Geometry: final body of the model. Coordinates: model frame, mm. Coordinates: 2 decimals unless noted, no trailing zeros. Order: outer loops, then holes, each group sorted by start corner. A loop starts at its lowest first (then second) coordinate and runs counter-clockwise, first axis right, second up. Notation, with made-up numbers: (72.5, 35) -> (103.5, 35) arc R13 ccw to (103.5, 39) -> close; hole circle Ø10 at (-5, -22). An arc over 180 degrees is marked (long way). Answer in a Markdown table with one row per item. Add a question column.
1) Ray query, line 1 (Y direction, x = 3.5, z = 0); line 2 (Y direction, x = 1.65, z = 0); line 3 (Y direction, x = 2.05, z = -2.5). Return the intervals inside material, ascending. Write a range as from..to.
2) Section query C-C on y = -41. Return the cut outline in (x, z), then the cut area to 3 significant figures.
3) Section query B-B on z = 0. Return the cut outline in (x, y), then the cut area to 4 significant figures.
4) Section query D-D on y = 33. Return the cut outline in (x, z), then the cut area to 3 significant figures.
5) Contact query for flat-ended pins moving along their axis: P1, Ø6, axis at y = 31, z = 1.5, coming from the +X side; P2, Ø14, axis at y = 33, z = 0, coming from the +X side. Output: stop coordinate, or through.
6) Section query A-A on x = 1.65. Return the cut outline in (y, z).
```python
from build123d import *

# Parameters (mm, degrees)
SKETCH1_W           = 43
SKETCH1_H           = 90
BOSS_EXTRUDE1_DEPTH = 6
CUT_EXTRUDE1_REACH  = 52.232
SKETCH2_R           = 2
CUT_EXTRUDE2_REACH  = 52.232
SKETCH3_R           = 4.1
FILLET1_R           = 20
SKETCH4_R           = 6
CUT_EXTRUDE3_DEPTH  = 3.5


with BuildPart() as part:
    # Sketch1 → Boss-Extrude1 (new body)
    with BuildSketch(Plane(origin=(0, 0, 0), x_dir=(0, 0, -1), z_dir=(1, 0, 0))):
        Rectangle(SKETCH1_W, SKETCH1_H)
    extrude(amount=BOSS_EXTRUDE1_DEPTH)

    # Sketch2 → Cut-Extrude1 (cut, up to next)
    with BuildSketch(Plane(origin=(6, 0, 0), x_dir=(0, 0, -1), z_dir=(1, 0, 0)), mode=Mode.PRIVATE) as cut_extrude1_sk1:
        with Locations((0, -41)):
            Circle(SKETCH2_R)
    cut_extrude1_tool1 = extrude(cut_extrude1_sk1.sketch, amount=-CUT_EXTRUDE1_REACH, mode=Mode.PRIVATE) & part.part
    # Sketch2 → Cut-Extrude1 (cut, up to next)
    with BuildSketch(Plane(origin=(6, 0, 0), x_dir=(0, 0, -1), z_dir=(1, 0, 0)), mode=Mode.PRIVATE) as cut_extrude1_sk2:
        with Locations((10, -41)):
            Circle(SKETCH2_R)
    cut_extrude1_tool2 = extrude(cut_extrude1_sk2.sketch, amount=-CUT_EXTRUDE1_REACH, mode=Mode.PRIVATE) & part.part
    # Sketch2 → Cut-Extrude1 (cut, up to next)
    with BuildSketch(Plane(origin=(6, 0, 0), x_dir=(0, 0, -1), z_dir=(1, 0, 0)), mode=Mode.PRIVATE) as cut_extrude1_sk3:
        with Locations((-10, -41)):
            Circle(SKETCH2_R)
    cut_extrude1_tool3 = extrude(cut_extrude1_sk3.sketch, amount=-CUT_EXTRUDE1_REACH, mode=Mode.PRIVATE) & part.part
    add(cut_extrude1_tool1.solids().sort_by_distance((6, -41, 0))[0], mode=Mode.SUBTRACT)
    add(cut_extrude1_tool2.solids().sort_by_distance((6, -41, -10))[0], mode=Mode.SUBTRACT)
    add(cut_extrude1_tool3.solids().sort_by_distance((6, -41, 10))[0], mode=Mode.SUBTRACT)

    # Sketch3 → Cut-Extrude2 (cut, up to next)
    with BuildSketch(Plane(origin=(6, 0, 0), x_dir=(0, 0, -1), z_dir=(1, 0, 0)), mode=Mode.PRIVATE) as cut_extrude2_sk1:
        with Locations((0, 33)):
            Circle(SKETCH3_R)
    cut_extrude2_tool1 = extrude(cut_extrude2_sk1.sketch, amount=-CUT_EXTRUDE2_REACH, mode=Mode.PRIVATE) & part.part
    add(cut_extrude2_tool1.solids().sort_by_distance((6, 33, 0))[0], mode=Mode.SUBTRACT)

    # Fillet1
    fillet1_edges = [part.edges().sort_by_distance(p)[0] for p in [
        (3, 45, 21.5),
        (3, 45, -21.5),
    ]]
    fillet(fillet1_edges, radius=FILLET1_R)

    # Sketch4 → Cut-Extrude3 (cut)
    with BuildSketch(Plane(origin=(6, 0, 0), x_dir=(0, 0, -1), z_dir=(1, 0, 0))):
        with Locations((0, 33)):
            Circle(SKETCH4_R)
    extrude(amount=-CUT_EXTRUDE3_DEPTH, mode=Mode.SUBTRACT)


solid = part.part
```
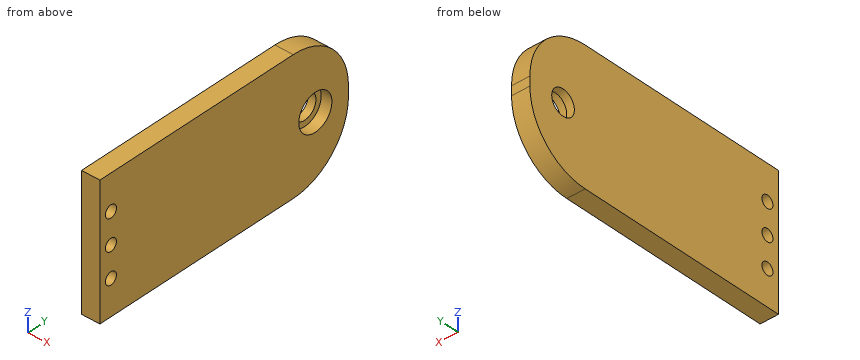
Result:
| question | item | result |
|---|---|---|
| 1 | line 1 | -45..-43, -39..27, 39..45 |
| 1 | line 2 | -45..-43, -39..28.9, 37.1..45 |
| 1 | line 3 | -45..29.75, 36.25..44.97 |
| 2 | outline | (0, -21.5) -> (6, -21.5) -> (6, -12) -> (0, -12) -> close; (0, -8) -> (6, -8) -> (6, -2) -> (0, -2) -> close; (0, 2) -> (6, 2) -> (6, 8) -> (0, 8) -> close; (0, 12) -> (6, 12) -> (6, 21.5) -> (0, 21.5) -> close |
| 2 | area | 186 mm2 |
| 3 | outline | (0, -45) -> (6, -45) -> (6, -43) -> (0, -43) -> close; (0, -39) -> (6, -39) -> (6, 27) -> (2.5, 27) -> (2.5, 28.9) -> (0, 28.9) -> close; (0, 37.1) -> (2.5, 37.1) -> (2.5, 39) -> (6, 39) -> (6, 45) -> (0, 45) -> close |
| 3 | area | 453.5 mm2 |
| 4 | outline | (0, -19.83) -> (6, -19.83) -> (6, -6) -> (2.5, -6) -> (2.5, -4.1) -> (0, -4.1) -> close; (0, 4.1) -> (2.5, 4.1) -> (2.5, 6) -> (6, 6) -> (6, 19.83) -> (0, 19.83) -> close |
| 4 | area | 175 mm2 |
| 5 | P1 | x = 2.5 |
| 5 | P2 | x = 6 |
| 6 | outline | (-45, -21.5) -> (25, -21.5) arc R20 ccw to (45, -1.5) -> (45, 1.5) arc R20 ccw to (25, 21.5) -> (-45, 21.5) -> close; hole circle Ø4 at (-41, -10); hole circle Ø4 at (-41, 0); hole circle Ø4 at (-41, 10); hole circle Ø8.2 at (33, 0) |
